from build123d import *

# Parameters (mm, degrees)
SKETCH_2_W              = 60
SKETCH_2_H              = 40
SKETCH_2_W_2            = 52
SKETCH_2_H_2            = 32
EXTRUDE_3_DEPTH         = 50
EXTRUDE_3_DEPTH_BACK    = 50
HOLE_WIZARD_5_5_5_5_1_D = 5.5


with BuildPart() as part:
    # Sketch 2 → Extrude 3 (new body, two sides)
    with BuildSketch(Plane.XY) as extrude_3_sk:
        Rectangle(SKETCH_2_W, SKETCH_2_H)
        Rectangle(SKETCH_2_W_2, SKETCH_2_H_2, mode=Mode.SUBTRACT)
    extrude(amount=EXTRUDE_3_DEPTH)
    extrude(extrude_3_sk.sketch, amount=-EXTRUDE_3_DEPTH_BACK)

    # Hole Wizard 5.5 _5.5_1 (through all)
    with Locations(Plane.ZY.offset(30)):
        with Locations((-33, 8), (-33, -8), (33, 8), (33, -8)):
            Hole(HOLE_WIZARD_5_5_5_5_1_D / 2)


solid = part.part
The model under review builds one solid part; all positions refer to its coordinate system, in mm. A direction names the side the tool comes from. Round coordinates to 2 decimals unless told otherwise and drop trailing zeros. Loops run counter-clockwise (first coordinate to the right, second up) from the corner with the lowest first, then second, coordinate; pieces in that order, holes last. Notation, with made-up numbers: (29.5, 55) -> (46.5, 55) arc R31 cw to (46.5, 91) -> close; hole circle Ø4 at (-18, 86.5). An arc over 180 degrees is marked (long way). Write item = value, one per line. Start each with the question number.
Item 1: Take a section at D-D on z = 33. Give the boundary of the cut face in (x, y), plus the area to 3 significant figures.
Item 2: Take a section at B-B on z = -29. Give the boundary of the cut face in (x, y).
Item 3: Mouldability with a two-part tool opening along Y and no side actions: class faces 1 (the cylindrical face through (-27.972, 8.121, -30.253)), 2 (the flat face through (0, -17, 50)), 3 (the flat face through (0, 20, 1)) as released by +Y, released by -Y, zero draft, split by the parting line, or undercut.
Item 4: Take a section at A-A on y = 14. Give the boundary of the cut face in (x, z), plus the area to 3 significant figures.
Item 5: Insertion check: pin 1 (7 mm diameter, centred on y = -8, z = 33, fed in from -X). The pin has a flat end and moves straight along its axis. Give the tip position at first contact, or say it passes through.
Item 6: To check wall thickness, follow L1, parallel to Y at x = -28, z = -33; L2, parallel to X at y = -10.5, z = -24.5; L3, parallel to Y at x = -5, z = 34. State the ranges of each line that lie inside material, in increasing order.
Item 7: For faces 4 (the flat face through (-30, 0, 1)), 5 (the flat face through (26, 0, 1)), list the 3-axis set-ups (+Z, -Z, +X, -X, +Y, -Y) from which the entire face can be reached by the end or side of a thin tool; tool diameter is ignored.
Item 8: Take a section at C-C on x = -16. Give the boundary of the cut face in (y, z).
Result:
q1.outline = (-30, -20) -> (30, -20) -> (30, -10.75) -> (26, -10.75) -> (26, -16) -> (-26, -16) -> (-26, -10.75) -> (-30, -10.75) -> close; (-30, -5.25) -> (-26, -5.25) -> (-26, 5.25) -> (-30, 5.25) -> close; (-30, 10.75) -> (-26, 10.75) -> (-26, 16) -> (26, 16) -> (26, 10.75) -> (30, 10.75) -> (30, 20) -> (-30, 20) -> close; (26, -5.25) -> (30, -5.25) -> (30, 5.25) -> (26, 5.25) -> close
q1.area = 648 mm²
q2.outline = (-30, -20) -> (30, -20) -> (30, 20) -> (-30, 20) -> close; hole (-26, -16) -> (26, -16) -> (26, 16) -> (-26, 16) -> close
q3.face_1 = undercut
q3.face_2 = zero draft
q3.face_3 = released by +Y
q4.outline = (-30, -50) -> (-26, -50) -> (-26, 50) -> (-30, 50) -> close; (26, -50) -> (30, -50) -> (30, 50) -> (26, 50) -> close
q4.area = 800 mm²
q5.pin_1 = -30
q6.L1 = -20 to -10.75, -5.25 to 5.25, 10.75 to 20
q6.L2 = -30 to -26, 26 to 30
q6.L3 = -20 to -16, 16 to 20
q7.face_4 = +Z, -Z, -X, +Y, -Y
q7.face_5 = +Z, -Z
q8.outline = (-20, -50) -> (-16, -50) -> (-16, 50) -> (-20, 50) -> close; (16, -50) -> (20, -50) -> (20, 50) -> (16, 50) -> close
